Can you work these out from the model? Positions are in its coordinate system, mm. Face numbers are marked on the shaded views. Round coordinates to 2 decimals unless told otherwise and drop trailing zeros. Loops run counter-clockwise (first coordinate to the right, second up) from the corner with the lowest first, then second, coordinate; pieces in that order, holes last.
(1) Thinking about a two-plate mould opening in X: for the marked faces 1 and 2, which applies, released by +X, released by -X, zero draft, split by the parting line, or undercut?
(2) I want a section at C-C on y = 1.5. Write out the boundary of the cut face in (x, z).
(3) If I drill on line 1 along Y through (x, z) = (1, 21); line 2 along Z through (x, y) = (-5, 7.5); line 3 along X through (y, z) = (1.25, -3.5), over which ranges is the centre line in solid material (lowest first)?
(4) I want a section at A-A on x = 0. Write out the boundary of the cut face in (y, z), plus the area to 3 significant figures.
(5) I want a section at B-B on y = 5. Write out the boundary of the cut face in (x, z), plus the area to 3 significant figures.
(6) Will these pins go through, and if not, where does the flat tip stop? pin 1 Ø0.5 at (y, z) = (14, 19.5) entering from -X; pin 2 Ø6 at (y, z) = (11.5, -1) entering from -X; pin 3 Ø1.8 at (x, y) = (5, 5) entering from -Z.
(7) I want a section at D-D on x = -5. Give the number of separate pieces and of enclosed holes in the cut face, plus the area to 3 significant figures.
from build123d import *

# Parameters (mm, degrees)
CUT_EXTRUDE1_REACH       = 2.3
SKETCH4_R                = 7.75
BOSS_EXTRUDE1_START      = 18
SKETCH13_W               = 2
SKETCH13_H               = 1.751149917
BOSS_EXTRUDE1_DEPTH      = 3
BOSS_EXTRUDE1_DEPTH_BACK = 2
SKETCH14_R               = 1
BOSS_EXTRUDE2_DEPTH      = 5
BOSS_EXTRUDE2_DEPTH_BACK = 7
SKETCH15_R               = 0.75
CUT_EXTRUDE2_DEPTH       = 15
SKETCH16_R               = 1
CUT_EXTRUDE3_DEPTH       = 20


with BuildPart() as part:
    # Sketch3 → Revolve1 (revolve)
    with BuildSketch(Plane.XY):
        Polygon((8.400325033, 0), (21.601834058, 18.8537088), (21.192258036, 19.140497019), (8, 0.3), (0, 0.3), (0, 0), align=None)
    revolve(axis=Axis((0, 0, 0), (0, 1, 0)))

    # Sketch4 → Cut-Extrude1 (cut, up to next)
    with BuildSketch(Plane(origin=(0, 0.3, 0), x_dir=(1, 0, 0), z_dir=(0, 1, 0)), mode=Mode.PRIVATE) as cut_extrude1_sk1:
        Circle(SKETCH4_R)
    cut_extrude1_tool1 = extrude(cut_extrude1_sk1.sketch, amount=-CUT_EXTRUDE1_REACH, mode=Mode.PRIVATE) & part.part
    add(cut_extrude1_tool1.solids().sort_by_distance((0, 0.3, 0))[0], mode=Mode.SUBTRACT)

    # Sketch13 → Boss-Extrude1 (add, two sides)
    with BuildSketch(Plane.XY.offset(BOSS_EXTRUDE1_START)) as boss_extrude1_sk:
        with Locations((0, 13.978133842)):
            Rectangle(SKETCH13_W, SKETCH13_H)
    extrude(amount=BOSS_EXTRUDE1_DEPTH)
    extrude(boss_extrude1_sk.sketch, amount=-BOSS_EXTRUDE1_DEPTH_BACK)

    # Sketch14 → Boss-Extrude2 (add, two sides)
    with BuildSketch(Plane.ZY.offset(1)) as boss_extrude2_sk:
        with Locations((21, 13.978133842)):
            Circle(SKETCH14_R)
    extrude(amount=BOSS_EXTRUDE2_DEPTH)
    extrude(boss_extrude2_sk.sketch, amount=-BOSS_EXTRUDE2_DEPTH_BACK)

    # Sketch15 → Cut-Extrude2 (cut)
    with BuildSketch(Plane.ZY.offset(6)):
        with Locations((21, 13.978133842)):
            Circle(SKETCH15_R)
    extrude(amount=-CUT_EXTRUDE2_DEPTH, mode=Mode.SUBTRACT)

    # Sketch16 → Cut-Extrude3 (cut)
    with BuildSketch(Plane.XY):
        with Locations((-5, 5)):
            Circle(SKETCH16_R)
        with Locations((5, 5)):
            Circle(SKETCH16_R)
    extrude(amount=CUT_EXTRUDE3_DEPTH, mode=Mode.SUBTRACT)


solid = part.part
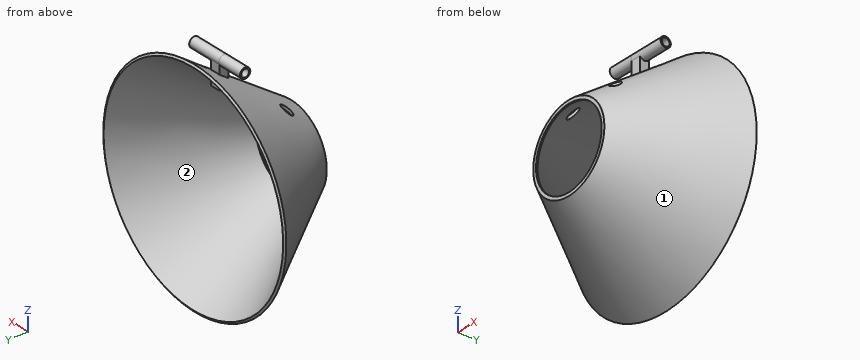
Filled sheet:
1. face 1: split by the parting line
1. face 2: undercut
2. outline: circle Ø18.9 at (0, 0); hole circle Ø17.68 at (0, 0)
3. line 1: y = 12.98 to 13.23, 14.73 to 14.98, 18.03 to 18.9
3. line 2: z = -12.7 to -12.04, 12.04 to 12.7
3. line 3: x = -8.59 to -7.93, 7.93 to 8.59
4. outline: (0, -8.4) - (18.85, -21.6) - (19.14, -21.19) - (0.3, -8) - (0.3, -7.75) - (0, -7.75) - close; (0, 7.75) - (0.3, 7.75) - (0.3, 8) - (13.1, 16.96) - (13.1, 16) - (14.85, 16) - (14.85, 18.19) - (19.14, 21.19) - (18.85, 21.6) - (14.85, 18.8) - (14.85, 20.52) arc R1 ccw (long way) to (13.1, 20.52) - (13.1, 17.57) - (0, 8.4) - close; hole circle Ø1.5 at (13.98, 21)
4. area: 30.8 mm2
5. outline: (-6, 9.56) - (-6, 10.28) arc R11.9 ccw (long way) to (6, 10.28) - (6, 9.56) arc R11.29 cw (long way) to start; (-4, 10.56) arc R11.29 cw to (4, 10.56) - (4, 11.21) arc R11.9 ccw to (-4, 11.21) - close
5. area: 41.8 mm2
6. pin 1: stops at x = -1
6. pin 2: stops at x = -18.53
6. pin 3: stops at z = -11.59
7. separate pieces: 4
7. enclosed holes: 1
7. area: 25.3 mm2
